Read the model definition and answer for the solid it produces. Units are mm, in the model's axes. Coordinates: 2 decimals unless noted, no trailing zeros. Loops run counter-clockwise (first coordinate to the right, second up) from the corner with the lowest first, then second, coordinate; pieces in that order, holes last. Notation, with made-up numbers: (23, 18) -> (75, 18) arc R21 cw to (75, 35) -> close; hole circle Ø5 at (-32, 86.5). An arc over 180 degrees is marked (long way). Answer as a JSON object with one key per item and string values. Group by question number.
1) Section B-B, the plane x = -36 is taken. Give the vertices of the cut face in (y, z), plus the area to 3 significant figures.
2) Section A-A, the plane x = -7 is taken. Give the vertices of the cut face in (y, z).
3) Consider probe 1 along Y at (x, z) = (-11, 1.35); probe 2 along X at (y, z) = (-5.75, 1.65); probe 3 along X at (y, z) = (-6.75, 1.35). Determine where each line is inside the solid, lowest interval first. Write a range as [from, to].
4) Section D-D, the plane z = 0.45 is taken. Count the separate pieces of the cut face and the enclosed holes in it, plus the area to 3 significant figures.
5) Section C-C, the plane x = -28.95 is taken. Give the vertices of the cut face in (y, z).
6) Flat-ended cylindrical pins translate along their axes: P1, Ø1.5, axis at y = -1.5, z = 1.5, coming from the -X side; P2, Ø2, axis at x = -54.5, y = -10.5, coming from the -Z side; P3, Ø1.6, axis at y = -13.5, z = 1, coming from the +X side; P4, Ø0.9, axis at x = -36.5, z = 1.5, coming from the -Y side. Find the tip coordinate at first contact, or state that the pin passes through.
Autodesk Inventor part; units mm, degrees
ref_plane "YZ Plane" through (0, 0, 0) normal (1, 0, 0) x (0, 1, 0)
ref_plane "XZ Plane" through (0, 0, 0) normal (0, 1, 0) x (-1, 0, 0)
ref_plane "XY Plane" through (0, 0, 0) normal (0, 0, 1) x (1, 0, 0)
sketch "スケッチ1" plane through (0, 0, 0) normal (0, 0, 1) x (1, 0, 0)
  line L0 (0, 0) -> (0, -3)
  line L1 (0, 0) -> (-15, 0)
  line L2 (-15, 0) -> (-15, -3)
  line L3 (-15, -3) -> (-30, -3)
  line L4 (-30, -3) -> (-30, 0)
  line L5 (-30, 0) -> (-45, 0)
  line L6 (-45, 0) -> (-45, -3)
  line L7 (-257.4775, 0) -> (-66.4062, 0)
  line L8 (-66.4062, 0) -> (-51.9242, -3.906)
  line L9 (-257.4775, 0) -> (-257.4775, -3)
  line L10 (-257.4775, -3) -> (-68.9626, -6)
  line L11 (-68.9626, -6) -> (-58.5737, -15.799)
  circle A0 centre (-53.7535, -10.6886) radius 4.025
  circle A1 centre (-53.7535, -10.6886) radius 1.5
  line L12 (0, -3) -> (0, -9)
  arc A2 (-54.2694, -3.6826) -> (-51.0532, -17.1739) centre (-53.7535, -10.6886) ccw
  line L13 (-54.2694, -3.6826) -> (-45, -3)
  line L14 (-51.0532, -17.1739) -> (-31.4218, -9)
  line L15 (-31.4218, -9) -> (0, -9)
  arc A3 (-46.7293, -10.7926) -> (-42.5418, -13.63) centre (-43.7046, -10.8374) ccw
  circle A4 centre (-43.7046, -10.8374) radius 1.5
  line L16 (-54.6828, -17.6519) -> (-41.7856, -19.3732)
  arc A5 (-41.7856, -19.3732) -> (-42.5418, -13.63) centre (-41.3887, -16.3996) ccw
  arc A6 (-58.5737, -15.799) -> (-54.6828, -17.6519) centre (-53.7535, -10.6886) ccw
  arc A7 (-46.7293, -10.7926) -> (-51.9242, -3.906) centre (-53.7535, -10.6886) ccw
  line L17 (-42, -3) -> (-33, -3)
  line L18 (-33, -3) -> (-33, -6)
  line L19 (-33, -6) -> (-42, -6)
  line L20 (-42, -6) -> (-42, -3)
  line L21 (-12, -3) -> (-3, -3)
  line L22 (-3, -3) -> (-3, -6)
  line L23 (-3, -6) -> (-12, -6)
  line L24 (-12, -6) -> (-12, -3)
  circle A8 centre (-40.95, -3) radius 1.05
  circle A9 centre (-34.05, -3) radius 1.05
  circle A10 centre (-34.05, -6) radius 1.05
  circle A11 centre (-40.95, -6) radius 1.05
  circle A12 centre (-10.95, -3) radius 1.05
  circle A13 centre (-4.05, -3) radius 1.05
  circle A14 centre (-4.05, -6) radius 1.05
  circle A15 centre (-10.95, -6) radius 1.05
  circle A16 centre (-28.95, -3) radius 1.05
  circle A17 centre (-16.05, -3) radius 1.05
  circle A18 centre (-41.3887, -16.3996) radius 1.25
  line L25 (-15.5802, -9) -> (-15.5802, -14)
  line L26 (-15.5802, -14) -> (-4.3492, -14)
  line L27 (-4.3492, -14) -> (-4.3492, -12)
  line L28 (-4.3492, -12) -> (-11.5802, -12)
  arc A19 (-11.5802, -9) -> (-11.5802, -12) centre (-11.5802, -10.5) ccw
  point P0 (-5.1, -6)
  point P1 (-9.9, -6)
  point P2 (-9.9, -3)
  point P3 (-5.1, -3)
  point P4 (-35.1, -6)
  point P5 (-39.9, -6)
  point P6 (-39.9, -3)
  point P7 (-35.1, -3)
  point P8 (-17.1, -3)
  point P9 (-27.9, -3)
  dimension "d0" = 3
  dimension "d1" = 15
  dimension "d2" = 3
  dimension "d3" = 15
  dimension "d5" = 15
  dimension "d6" = 3
  dimension "d7" = 3
  dimension "d8" = 8.05
  dimension "d10" = 3
  dimension "d11" = 6
  dimension "d12" = 6
  dimension "d13" = 6.05
  dimension "d14" = 3
  dimension "d15" = 9
  dimension "d16" = 3
  dimension "d17" = 9
  dimension "d18" = 3
  dimension "d19" = 3
  dimension "d20" = 3
  dimension "d21" = 3
  dimension "d22" = 3
  dimension "d23" = 3
  dimension "d24" = 2.1
  dimension "d25" = 2.1
  dimension "d26" = 2.1
  dimension "d27" = 2.1
  dimension "d28" = 2.1
  dimension "d29" = 2.1
  dimension "d30" = 2.1
  dimension "d31" = 2.1
  dimension "d32" = 2.1
  dimension "d33" = 2.1
  dimension "d34" = 2.5
  dimension "d36" = 3
  dimension "d37" = 3
  dimension "d38" = 2
  dimension "d39" = 4
extrude "押し出し1" add sketch "スケッチ1" along normal blind 3 contours L0 L12 L15 L14 A3 A7 L8 L13 L6 L5 L4 A16 L3 A17 L2 L1 | A19 L28 L27 L26 L25 L15 | L14 A2 L13 L8 A7 A3 | A0
properties part number "シールド先端接続"
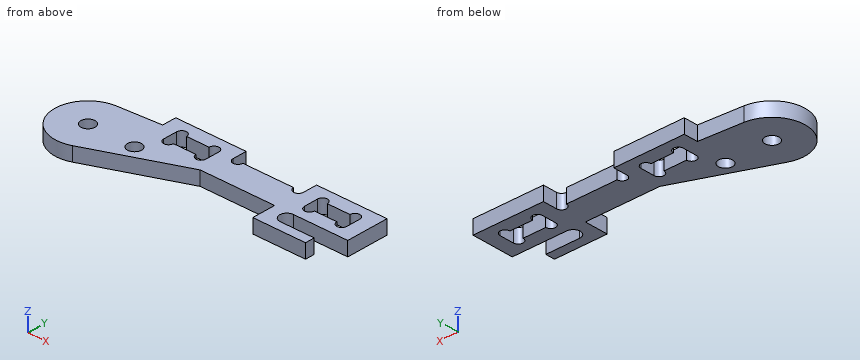
Determined:
{
 "1": {"outline": "(-10.91, 0) -> (-6, 0) -> (-6, 3) -> (-10.91, 3) -> close; (-3, 0) -> (0, 0) -> (0, 3) -> (-3, 3) -> close", "area": "23.7 mm²"},
 "2": {"outline": "(-14, 0) -> (-12, 0) -> (-12, 3) -> (-14, 3) -> close; (-9, 0) -> (-6, 0) -> (-6, 3) -> (-9, 3) -> close; (-3, 0) -> (0, 0) -> (0, 3) -> (-3, 3) -> close"},
 "3": {"probe 1": "[-14, -12], [-9, -7.05], [-1.95, 0]", "probe 2": "[-58.75, -42], [-33, -12], [-3, 0]", "probe 3": "[-59.57, -41.68], [-40.22, -34.78], [-33.32, -11.68], [-10.22, -4.78], [-3.32, 0]"},
 "4": {"separate pieces": "1", "enclosed holes": "4", "area": "536 mm²"},
 "5": {"outline": "(-9, 0) -> (-4.05, 0) -> (-4.05, 3) -> (-9, 3) -> close"},
 "6": {"P1": "x = -45", "P2": "z = 0", "P3": "x = -4.35", "P4": "y = -11.3"}
}
